```python
from build123d import *

# Parameters (mm, degrees)
F1_DEPTH = 1060
F2_R     = 2


with BuildPart() as f1:
    # F0 (on Front) → F1 (new body)
    with BuildSketch(Plane.XZ):
        with BuildLine():
            Line((5.301232, 14.000001), (-14.698768, 14.000001))
            ThreePointArc((-14.698768, 14.000001), (-18.234301, 12.535535), (-19.698768, 9.000001))
            Line((-19.698768, 9.000001), (-19.698768, -30.999999))
            ThreePointArc((-19.698768, -30.999999), (-18.234301, -34.535533), (-14.698768, -35.999999))
            Line((-14.698768, -35.999999), (5.301232, -35.999999))
            Line((5.301232, -35.999999), (25.301232, -35.999999))
            ThreePointArc((25.301232, -35.999999), (28.836766, -34.535533), (30.301232, -30.999999))
            Line((30.301232, -30.999999), (30.301232, 9.000001))
            ThreePointArc((30.301232, 9.000001), (28.836766, 12.535535), (25.301232, 14.000001))
            Line((25.301232, 14.000001), (5.301232, 14.000001))
        make_face()
        Polygon((-15.698768, -31.999999), (-15.698768, 10.000001), (5.301232, 10.000001), (26.301232, 10.000001), (26.301232, -31.999999), (5.301232, -31.999999), align=None, mode=Mode.SUBTRACT)
    extrude(amount=F1_DEPTH)

    # F2
    f2_edges = [f1.edges().sort_by_distance(p)[0] for p in [
        (-15.698768, -530, 10.000001),
        (26.301232, -530, 10.000001),
        (26.301232, -530, -31.999999),
        (-15.698768, -530, -31.999999),
    ]]
    fillet(f2_edges, radius=F2_R)


solid = f1.part
```
The listing builds one solid part. Answer for the finished solid, in the listing's coordinates (mm). A direction names the side the tool comes from. Give positions to 0.01 mm unless a question says otherwise; leave off trailing zeros. Order: outer loops, then holes, each group sorted by start corner. A loop starts at its lowest first (then second) coordinate and runs counter-clockwise, first axis right, second up.
Item 1: The part is cut by section A-A, the plane z = -8. Give the vertices of the cut face in (x, y), and give its area (3 significant figures).
From the geometry:
outline: (-19.7, -1060) - (-15.7, -1060) - (-15.7, 0) - (-19.7, 0) - close; (26.3, -1060) - (30.3, -1060) - (30.3, 0) - (26.3, 0) - close
area: 8,480 mm2
Item 2: The part is cut by section C-C, the plane y = -688.5. Give the vertices of the cut face in (x, z), and give its area (3 significant figures).
From the geometry:
outline: (-19.7, -31) arc R5 ccw to (-14.7, -36) - (25.3, -36) arc R5 ccw to (30.3, -31) - (30.3, 9) arc R5 ccw to (25.3, 14) - (-14.7, 14) arc R5 ccw to (-19.7, 9) - close; hole (-15.7, -30) arc R2 ccw to (-13.7, -32) - (24.3, -32) arc R2 ccw to (26.3, -30) - (26.3, 8) arc R2 ccw to (24.3, 10) - (-13.7, 10) arc R2 ccw to (-15.7, 8) - close
area: 718 mm2
Item 3: The part is cut by section B-B, the plane x = 12. Give the vertices of the cut face in (y, z).
From the geometry:
outline: (-1060, -36) - (0, -36) - (0, -32) - (-1060, -32) - close; (-1060, 10) - (0, 10) - (0, 14) - (-1060, 14) - close
Item 4: For a pull along X with two mould halves and no side action, classify faces 1 (the face through (30.301, -523, -11)), 2 (the face through (27, -1060, -11)), 3 (the face through (5, -523, 10)) as pulls with the +X half, pulls with the -X half, needs draft (parallel to the pull), parting line crosses it, or undercut.
From the geometry:
face 1: pulls with the +X half
face 2: needs draft
face 3: undercut
Item 5: Which of the six approach directions +Z, -Z, +X, -X, +Y, -Y give full straight-line access (tool end or side, diameter ignored) to faces 4 (the face through (-15.699, -523, -11)), 5 (the face through (-19.699, -523, -11))?
From the geometry:
face 4: +Y, -Y
face 5: +Z, -Z, -X, +Y, -Y
Item 6: Find the intervals of material crossed by probe 1 along Z at (x, y) = (23, -430); probe 2 along Z at (x, y) = (25, -186); probe 3 along X at (y, z) = (-52, -24), in increasing order.
From the geometry:
probe 1: z = -36 to -32, 10 to 14
probe 2: z = -36 to -31.87, 9.87 to 14
probe 3: x = -19.7 to -15.7, 26.3 to 30.3
